Part model, mm, in its own coordinate system. A direction names the side the tool comes from. Coordinates: 2 decimals unless noted, no trailing zeros. Loops run counter-clockwise (first coordinate to the right, second up) from the corner with the lowest first, then second, coordinate; pieces in that order, holes last. Notation, with made-up numbers: (46.5, 58.5) -> (101.5, 58.5) arc R20 cw to (101.5, 67.5) -> close; hole circle Ø6 at (86, 69.5). An arc over 180 degrees is marked (long way). One line per item, written item: value. Start each with the question number.
from build123d import *

# Parameters (mm, degrees)
SKETCH1_W                = 50
SKETCH1_H                = 100
BOSS_EXTRUDE1_DEPTH      = 0.9125
BOSS_EXTRUDE1_DEPTH_BACK = 0.9125


with BuildPart() as part:
    # Sketch1 → Boss-Extrude1 (new body, two sides)
    with BuildSketch(Plane(origin=(0, 0, 0), x_dir=(1, 0, 0), z_dir=(0, 1, 0))) as boss_extrude1_sk:
        Rectangle(SKETCH1_W, SKETCH1_H)
        with BuildLine():
            Line((4.7625, 35.2375), (4.7625, -35.2375))
            ThreePointArc((4.7625, -35.2375), (0, -40), (-4.7625, -35.2375))
            Line((-4.7625, -35.2375), (-4.7625, 35.2375))
            ThreePointArc((-4.7625, 35.2375), (0, 40), (4.7625, 35.2375))
        make_face(mode=Mode.SUBTRACT)
    extrude(amount=BOSS_EXTRUDE1_DEPTH)
    extrude(boss_extrude1_sk.sketch, amount=-BOSS_EXTRUDE1_DEPTH_BACK)


solid = part.part
1) Slice it at A-A (z = -24.5). Give the cut face in (x, y), then the cut area to 3 significant figures.
2) Slice it at B-B (x = 0). Give the cut face in (y, z).
3) Probe line 1 (X direction, y = -0.5, z = -30); line 2 (Z direction, x = 1.5, y = -0.6). List the from-to ranges inside material, lowest first. Write a range as from..to.
4) Pull direction Z, two halves, no side cores. Call faces 1 (the cylindrical face through (0, 0, 40)), 2 (the flat face through (5, 0.912, -1)), 3 (the flat face through (-4.762, 0, 0)), 4 (the flat face through (0, 0, -50)): +Z half, -Z half, draft (parallel to the pull), parting line (faces both ways), or undercut.
5) Tool access for faces 5 (the flat face through (25, 0, 1)), 6 (the flat face through (4.762, 0, 0)): list every direction of +Z, -Z, +X, -X, +Y, -Y with a clear straight run to the whole face (end or side of a thin tool).
6) Slice it at C-C (y = -0.1). Give the cut face in (x, z) (1 decimal).
Check sheet entries:
1. outline: (-25, -0.91) -> (-4.76, -0.91) -> (-4.76, 0.91) -> (-25, 0.91) -> close; (4.76, -0.91) -> (25, -0.91) -> (25, 0.91) -> (4.76, 0.91) -> close
1. area: 73.9 mm^2
2. outline: (-0.91, -50) -> (0.91, -50) -> (0.91, -40) -> (-0.91, -40) -> close; (-0.91, 40) -> (0.91, 40) -> (0.91, 50) -> (-0.91, 50) -> close
3. line 1: x = -25..-4.76, 4.76..25
3. line 2: z = -50..-39.76, 39.76..50
4. face 1: undercut
4. face 2: draft
4. face 3: undercut
4. face 4: -Z half
5. face 5: +Z, -Z, +X, +Y, -Y
5. face 6: +Y, -Y
6. outline: (-25, -50) -> (25, -50) -> (25, 50) -> (-25, 50) -> close; hole (-4.8, -35.2) arc R4.8 ccw to (4.8, -35.2) -> (4.8, 35.2) arc R4.8 ccw to (-4.8, 35.2) -> close
